Read the model definition and answer for the solid it produces. Units are mm, in the model's axes. A direction names the side the tool comes from. Coordinates: 2 decimals unless noted, no trailing zeros. Loops run counter-clockwise (first coordinate to the right, second up) from the corner with the lowest first, then second, coordinate; pieces in that order, holes last.
from build123d import *

# Parameters (mm, degrees)
ESBO_O2_W                = 51
ESBO_O2_H                = 50
RESSALTO_EXTRUS_O2_DEPTH = 6
CORTE_EXTRUS_O1_START    = -1
CORTE_EXTRUS_O1_DEPTH    = 15
PADR_OCIRCULAR1_COUNT    = 4


with BuildPart() as part:
    # Esboço2 → Ressalto-extrusão2 (new body)
    with BuildSketch(Plane(origin=(0, 0, 0), x_dir=(1, 0, 0), z_dir=(0, 1, 0))):
        Rectangle(ESBO_O2_W, ESBO_O2_H)
    extrude(amount=RESSALTO_EXTRUS_O2_DEPTH)

    # Esboço3 → Corte-extrusão1 (cut)
    with BuildSketch(Plane.ZY.offset(-25.5).offset(CORTE_EXTRUS_O1_START)):
        Polygon((-1.421809274, 1.180167117), (0.86511687, 0.858760608), (2.286926144, 2.678593491), (1.421809274, 4.819832883), (-0.86511687, 5.141239392), (-2.286926144, 3.321406509), align=None)
    corte_extrus_o1 = extrude(amount=CORTE_EXTRUS_O1_DEPTH, mode=Mode.SUBTRACT)

    # PadrãoCircular1: Corte-extrusão1 ×4 about axis
    padr_ocircular1_axis = Axis((0, 0, 0), (0, 1, 0))
    for i in range(1, PADR_OCIRCULAR1_COUNT):
        add(corte_extrus_o1.rotate(padr_ocircular1_axis, i * 360 / PADR_OCIRCULAR1_COUNT), mode=Mode.SUBTRACT)


solid = part.part
Q1. A cutting plane is placed at B-B (x = -18.5). Give the vertices of the cut face in (y, z), then the cut area to 3 significant figures.
Findings below:
outline: (0, -25) - (6, -25) - (6, 25) - (0, 25) - close; hole (0.86, -0.87) - (2.68, -2.29) - (4.82, -1.42) - (5.14, 0.87) - (3.32, 2.29) - (1.18, 1.42) - close
area: 286 mm2
Q2. Flat-ended cylindrical pins translate along their axes: pin 1 Ø1.3 at (x, y) = (-0.5, 2.5) entering from +Z; pin 2 Ø2 at (y, z) = (3.5, -0.5) entering from +X. Find the tip coordinate at first contact, or state that the pin passes through.
Findings below:
pin 1: stops at z = 11.5
pin 2: stops at x = 11.5
Q3. Which of the six approach directions +Z, -Z, +X, -X, +Y, -Y give full straight-line access (tool end or side, diameter ignored) to faces 1 (the face through (0, 0, 0)), 2 (the face through (-1.86, 3.73, 18.34)), 3 (the face through (-1.86, 2.27, -18.34)), 4 (the face through (-18.6, 4.2, 1.6)), 5 (the face through (-0.4, 0.3, 25))?
Findings below:
face 1: +Z, -Z, +X, -X, -Y
face 2: +Z
face 3: -Z
face 4: -X
face 5: +Z, +X, -X, +Y, -Y
Q4. A cutting plane is placed at A-A (z = 18). Give the vertices of the cut face in (x, y).
Findings below:
outline: (-25.5, 0) - (25.5, 0) - (25.5, 6) - (-25.5, 6) - close; hole (-2.29, 2.68) - (-0.87, 0.86) - (1.42, 1.18) - (2.29, 3.32) - (0.87, 5.14) - (-1.42, 4.82) - close
Q5. Determine the mould class of faces 6 (the face through (1.86, 2.27, 18.34)), 7 (the face through (18.6, 2.27, -1.86)), 8 (the face through (-0.4, 0.3, -25)) for opening direction Z: +Z half, -Z half, draft (parallel to the pull), parting line (faces both ways), or undercut.
Findings below:
face 6: draft
face 7: undercut
face 8: -Z half
Q6. A cutting plane is placed at C-C (z = 0). Give the vertices of the cut face in (x, y).
Findings below:
outline: (-25.5, 0) - (25.5, 0) - (25.5, 0.98) - (11.5, 0.98) - (11.5, 5.02) - (25.5, 5.02) - (25.5, 6) - (-25.5, 6) - (-25.5, 5.02) - (-11.5, 5.02) - (-11.5, 0.98) - (-25.5, 0.98) - close
Q7. Straight lines are drawn through the part: probe 1 along Z at (x, y) = (-1, 2.8); probe 2 along Y at (x, z) = (14, 0); probe 3 along Z at (x, y) = (-12.5, 3). For each, find the intervals that lie inside material, in ascending order.
Findings below:
probe 1: z = -11.5 to 11.5
probe 2: y = 0 to 0.98, 5.02 to 6
probe 3: z = -25 to -2.16, 2.16 to 25
